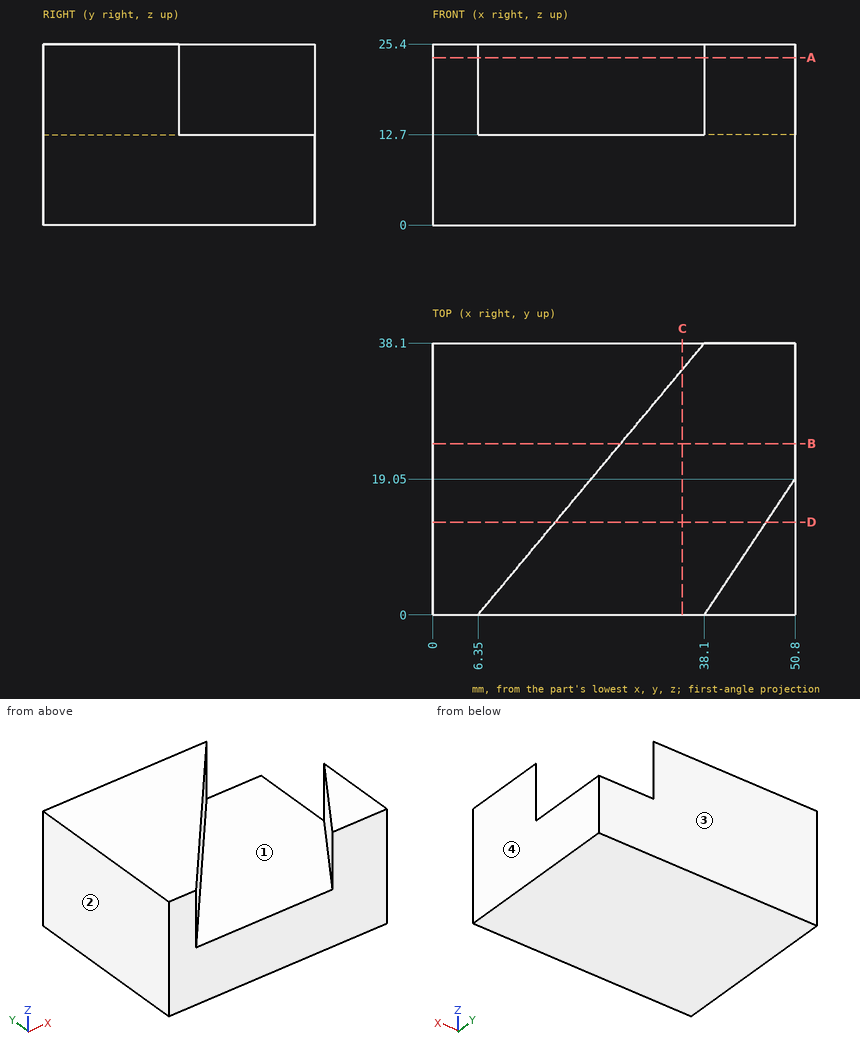
Answer from the drawing. Dimensions are ordinates in mm from the lowest x, y and z of the part. Give positions to 0.01 mm unless a question says otherwise; leave off trailing zeros. Write each loop counter-clockwise with the first axis right and the second up, starting at its lowest first coordinate (ties: lowest second). Pieces come first, ordered by that corner, then holes. Notation, with made-up numbers: (52, 66) -> (99, 66) arc R17 cw to (99, 74) -> close; hole circle Ø9 at (55, -17). An arc over 180 degrees is marked (long way). Use a Markdown table: item, result.
(1) Find the intervals of material crossed by probe 1 along Z at (x, y) = (48, 33); probe 2 along X at (y, z) = (9, 13.75); probe 3 along X at (y, z) = (36, 16.75), in increasing order. Write a range as from..to.
Return value:
| item | result |
|---|---|
| probe 1 | 0..12.7 |
| probe 2 | 0..13.85, 44.1..50.8 |
| probe 3 | 0..36.35 |
(2) Section D-D, the plane y = 13 is taken. Determine the outline of the cut face in (x, z).
Return value:
| item | result |
|---|---|
| outline | (0, 0) -> (50.8, 0) -> (50.8, 25.4) -> (46.77, 25.4) -> (46.77, 12.7) -> (17.18, 12.7) -> (17.18, 25.4) -> (0, 25.4) -> close |
(3) Section B-B, the plane y = 24 is taken. Determine the outline of the cut face in (x, z), then the cut area to 3 significant figures.
Return value:
| item | result |
|---|---|
| outline | (0, 0) -> (50.8, 0) -> (50.8, 12.7) -> (26.35, 12.7) -> (26.35, 25.4) -> (0, 25.4) -> close |
| area | 980 mm2 |
(4) Determine the mould class of the marked faces 1, 2, 3 and 4 for opening direction X: released by +X, released by -X, zero draft, split by the parting line, or undercut.
Return value:
| item | result |
|---|---|
| face 1 | undercut |
| face 2 | released by -X |
| face 3 | zero draft |
| face 4 | released by +X |
(5) Flat-ended cylindrical pins translate along their axes: P1, Ø1, axis at x = 40.5, y = 28.5, coming from the +Z side; P2, Ø1.5, axis at x = 29.5, z = 22.5, coming from the -Y side. Find the tip coordinate at first contact, or state that the pin passes through.
Return value:
| item | result |
|---|---|
| P1 | z = 12.7 |
| P2 | y = 26.88 |
(6) Section C-C, the plane x = 35 is taken. Determine the outline of the cut face in (y, z).
Return value:
| item | result |
|---|---|
| outline | (0, 0) -> (38.1, 0) -> (38.1, 25.4) -> (34.38, 25.4) -> (34.38, 12.7) -> (0, 12.7) -> close |
(7) Section A-A, the plane z = 23.5 is taken. Determine the outline of the cut face in (x, y), then the cut area to 3 significant figures.
Return value:
| item | result |
|---|---|
| outline | (0, 0) -> (6.35, 0) -> (38.1, 38.1) -> (0, 38.1) -> close; (38.1, 0) -> (50.8, 0) -> (50.8, 19.05) -> close |
| area | 968 mm2 |
